from build123d import *

# Parameters (mm, degrees)
F0_R     = 7.9375
F0_R_2   = 2.54
F1_DEPTH = 14.2875
F2_SIZE2 = 3.96875
F2_SIZE  = 1.5875
F3_R     = 6.35
F3_R_2   = 2.54
F4_DEPTH = 6.35


with BuildPart() as f1:
    # F0 (on Top) → F1 (new body)
    with BuildSketch(Plane.XY):
        Circle(F0_R)
        Circle(F0_R_2, mode=Mode.SUBTRACT)
    extrude(amount=F1_DEPTH)

    # F2
    f2_edges = [f1.edges().sort_by_distance(p)[0] for p in [
        (-7.9375, 0, 0),
    ]]
    chamfer(f2_edges, length=F2_SIZE, length2=F2_SIZE2)

    # F3 (on face) → F4 (cut)
    with BuildSketch(Plane.XY.offset(14.2875)):
        Circle(F3_R)
        Circle(F3_R_2, mode=Mode.SUBTRACT)
    extrude(amount=-F4_DEPTH, mode=Mode.SUBTRACT)


solid = f1.part
Verification items for the finished model (mm, model axes). Round coordinates to 2 decimals unless told otherwise and drop trailing zeros. Loops run counter-clockwise (first coordinate to the right, second up) from the corner with the lowest first, then second, coordinate; pieces in that order, holes last. Notation, with made-up numbers: (82.5, 40.25) - (130.5, 40.25) arc R28 cw to (130.5, 68.25) - close; hole circle Ø8 at (89, -17). An arc over 180 degrees is marked (long way). Answer in a Markdown table with one row per item. Add a question column.
Q1. Section check A-A on x = 0. Enter the section's corners in (y, z), plus the area to 3 significant figures.
Q2. Release check for a two-part mould opening along Y. For faces 1 (the face through (-3.302, -2.532, 0.077)), 2 (the face through (-1.38, -6.2, 11.16)), 3 (the face through (3, 0, 7.938)), 4 (the face through (0, 7, 14.288)) record: pulls with the +Y half, pulls with the -Y half, needs draft (parallel to the pull), parting line crosses it, or undercut.
Q3. Section check C-C on z = 7.5. Enter the section's corners in (x, y) (1 decimal).
Q4. Gauge pin test, flat ends, axial feed: pin 1 (1 mm diameter, centred on x = 4.5, z = 11.5, fed in from +Y); pin 2 (1.5 mm diameter, centred on y = 6, z = 10, fed in from +X); pin 3 (5 mm diameter, centred on y = -3, z = 10.5, fed in from -X). Record the tip position at first contact, or that the pin passes through.
Q5. Material ranges on line 1 (Y direction, x = 0, z = 8.5); line 2 (Y direction, x = 0, z = 2); line 3 (X direction, y = -5.75, z = 12.75), recorded low to high.
Found:
| question | item | result |
|---|---|---|
| 1 | outline | (-7.94, 1.59) - (-3.97, 0) - (-2.54, 0) - (-2.54, 7.94) - (-6.35, 7.94) - (-6.35, 14.29) - (-7.94, 14.29) - close; (2.54, 0) - (3.97, 0) - (7.94, 1.59) - (7.94, 14.29) - (6.35, 14.29) - (6.35, 7.94) - (2.54, 7.94) - close |
| 1 | area | 99.5 mm² |
| 2 | face 1 | parting line crosses it |
| 2 | face 2 | undercut |
| 2 | face 3 | undercut |
| 2 | face 4 | needs draft |
| 3 | outline | circle Ø15.9 at (0, 0); hole circle Ø5.1 at (0, 0) |
| 4 | pin 1 | stops at y = 6.86 |
| 4 | pin 2 | stops at x = 5.95 |
| 4 | pin 3 | stops at x = -7.92 |
| 5 | line 1 | y = -7.94 to -6.35, 6.35 to 7.94 |
| 5 | line 2 | y = -7.94 to -2.54, 2.54 to 7.94 |
| 5 | line 3 | x = -5.47 to -2.69, 2.69 to 5.47 |
